from build123d import *

# Parameters (mm, degrees)
SKETCH_1_W                         = 148
SKETCH_1_H                         = 90
SKETCH_1_R                         = 11
SKETCH_1_R_2                       = 2.65
SM_BASE_FLANGE_1_DEPTH             = 4
SM_EDGE_FLANGE_1_STRIP_W           = 24
SM_EDGE_FLANGE_1_STRIP_H           = 4
SM_EDGE_FLANGE_1_STRIP_CUT_DEPTH   = 90
SM_EDGE_FLANGE_1_STRIP_2_W         = 24
SM_EDGE_FLANGE_1_STRIP_2_H         = 4
SM_EDGE_FLANGE_1_STRIP_CUT_2_DEPTH = 90
SM_EDGE_FLANGE_1_DEPTH             = 90
SM_EDGE_FLANGE_1_BEND_DEPTH        = 90
SKETCH_12_R                        = 2
CUT_EXTRUDE_1_DEPTH                = 161.031246949
FILLET_1_R                         = 10
SKETCH_13_R                        = 2
CUT_EXTRUDE_2_DEPTH                = 96.822753039


# Sheet-metal steps are written as plain solids
with BuildPart() as part:
    # Sketch 1 → Базовая кромка1 (new body)
    with BuildSketch(Plane.XY):
        Rectangle(SKETCH_1_W, SKETCH_1_H)
        Circle(SKETCH_1_R, mode=Mode.SUBTRACT)
        with Locations((20, 0)):
            Circle(SKETCH_1_R_2, mode=Mode.SUBTRACT)
        with Locations((-20, 0)):
            Circle(SKETCH_1_R_2, mode=Mode.SUBTRACT)
        with BuildLine():
            Line((-4.9, -36.5), (-4.9, -39.5))
            ThreePointArc((-4.9, -39.5), (-7, -41.6), (-9.1, -39.5))
            Line((-9.1, -39.5), (-9.1, -36.5))
            ThreePointArc((-9.1, -36.5), (-7, -34.4), (-4.9, -36.5))
        make_face(mode=Mode.SUBTRACT)
        with BuildLine():
            Line((9.1, -36.5), (9.1, -39.5))
            ThreePointArc((9.1, -39.5), (7, -41.6), (4.9, -39.5))
            Line((4.9, -39.5), (4.9, -36.5))
            ThreePointArc((4.9, -36.5), (7, -34.4), (9.1, -36.5))
        make_face(mode=Mode.SUBTRACT)
    extrude(amount=-SM_BASE_FLANGE_1_DEPTH)

    # Ребро-кромка1 strip (across the edge) → Ребро-кромка1 strip cut (cut)
    with BuildSketch(Plane(origin=(-74, 45, 0), x_dir=(1, 0, 0), z_dir=(0, -1, 0))):
        with Locations((-4, -2)):
            Rectangle(SM_EDGE_FLANGE_1_STRIP_W, SM_EDGE_FLANGE_1_STRIP_H)
    extrude(amount=SM_EDGE_FLANGE_1_STRIP_CUT_DEPTH, mode=Mode.SUBTRACT)

    # Ребро-кромка1 strip 2 (across the edge) → Ребро-кромка1 strip cut 2 (cut)
    with BuildSketch(Plane(origin=(74, -45, 0), x_dir=(-1, 0, 0), z_dir=(0, 1, 0))):
        with Locations((-4, -2)):
            Rectangle(SM_EDGE_FLANGE_1_STRIP_2_W, SM_EDGE_FLANGE_1_STRIP_2_H)
    extrude(amount=SM_EDGE_FLANGE_1_STRIP_CUT_2_DEPTH, mode=Mode.SUBTRACT)

    # Ребро-кромка1 section (across the edge) → Ребро-кромка1 (add)
    with BuildSketch(Plane(origin=(-74, 45, 0), x_dir=(1, 0, 0), z_dir=(0, -1, 0))):
        with BuildLine():
            Line((0, 4), (0, 41))
            Line((0, 41), (4, 41))
            Line((4, 41), (4, 4))
            ThreePointArc((4, 4), (5.171572875, 1.171572875), (8, 0))
            Line((8, 0), (8, -4))
            ThreePointArc((8, -4), (2.343145751, -1.656854249), (0, 4))
        make_face()
    extrude(amount=SM_EDGE_FLANGE_1_DEPTH)

    # Ребро-кромка1 section 2 (across the edge) → Ребро-кромка1 bend (add)
    with BuildSketch(Plane(origin=(74, -45, 0), x_dir=(-1, 0, 0), z_dir=(0, 1, 0))):
        with BuildLine():
            Line((0, 4), (0, 41))
            Line((0, 41), (4, 41))
            Line((4, 41), (4, 4))
            ThreePointArc((4, 4), (5.171572875, 1.171572875), (8, 0))
            Line((8, 0), (8, -4))
            ThreePointArc((8, -4), (2.343145751, -1.656854249), (0, 4))
        make_face()
    extrude(amount=SM_EDGE_FLANGE_1_BEND_DEPTH)

    # Эскиз12 → Вырез-Вытянуть1 (cut, through all)
    with BuildSketch(Plane(origin=(74, 0, 0), x_dir=(0, 0, -1), z_dir=(1, 0, 0))):
        with Locations((-31, 35)):
            Circle(SKETCH_12_R)
        with Locations((-31, -35)):
            Circle(SKETCH_12_R)
        with Locations((-31, 0)):
            Circle(SKETCH_12_R)
    extrude(amount=-CUT_EXTRUDE_1_DEPTH, mode=Mode.SUBTRACT)

    # Скругление1
    fillet_1_edges = [part.edges().sort_by_distance(p)[0] for p in [
        (72, -45, 41),
        (72, 45, 41),
        (-72, 45, 41),
        (-72, -45, 41),
    ]]
    fillet(fillet_1_edges, radius=FILLET_1_R)

    # Эскиз13 → Вырез-Вытянуть2 (cut, through all)
    with BuildSketch(Plane.XY):
        with Locations((-32, 38)):
            Circle(SKETCH_13_R)
        with Locations((32, 38)):
            Circle(SKETCH_13_R)
        with Locations((32, -38)):
            Circle(SKETCH_13_R)
        with Locations((-32, -38)):
            Circle(SKETCH_13_R)
    extrude(amount=-CUT_EXTRUDE_2_DEPTH, mode=Mode.SUBTRACT)


solid = part.part
Check sheet for the modelled part. Datum: model origin and axes. Units: mm. A direction names the side the tool comes from. Coordinates: 2 decimals unless noted, no trailing zeros. Loops run counter-clockwise (first coordinate to the right, second up) from the corner with the lowest first, then second, coordinate; pieces in that order, holes last. Notation, with made-up numbers: (38.25, 54) -> (92.25, 54) arc R33 ccw to (92.25, 90) -> close; hole circle Ø3 at (8, -21.75). An arc over 180 degrees is marked (long way). Answer in a Markdown table with one row per item.
1. Sectioned sample at B-B, the plane z = 8. Record the boundary of the cut face in (x, y).
Check values:
| item | result |
|---|---|
| outline | (-74, -45) -> (-70, -45) -> (-70, 45) -> (-74, 45) -> close; (70, -45) -> (74, -45) -> (74, 45) -> (70, 45) -> close |
2. Material ranges on line 1 along Y through (x, z) = (71.7, 31); line 2 along Y through (x, z) = (-32, -1.5); line 3 along X through (y, z) = (-32, 27), recorded low to high. Write a range as [from, to].
Check values:
| item | result |
|---|---|
| line 1 | y = [-45, -37], [-33, -2], [2, 33], [37, 45] |
| line 2 | y = [-45, -40], [-36, 36], [40, 45] |
| line 3 | x = [-74, -70], [70, 74] |
3. Go/stop test with flat-tipped pins: pin 1 (2.5 mm diameter, centred on x = 32, y = 38, fed in from -Z); pin 2 (6.5 mm diameter, centred on x = 32, y = -38, fed in from -Z); pin 3 (2.5 mm diameter, centred on y = -37.5, z = -3, fed in from -X); pin 4 (8.5 mm diameter, centred on x = 20, y = 0, fed in from +Z). Record where each tip stops, or that it passes through.
Check values:
| item | result |
|---|---|
| pin 1 | passes through |
| pin 2 | stops at z = -4 |
| pin 3 | stops at x = -71.56 |
| pin 4 | stops at z = 0 |
4. Release check for a two-part mould opening along Y. For faces 4 (the face through (-68.859, 0.63, 1.203)), 5 (the face through (7, -34.4, -2)), 6 (the face through (0, -45, -1)), 7 (the face through (71.97, 42.15, 37.99)) record: released by +Y, released by -Y, zero draft, split by the parting line, or undercut.
Check values:
| item | result |
|---|---|
| face 4 | zero draft |
| face 5 | undercut |
| face 6 | released by -Y |
| face 7 | released by +Y |
5. Access from +Z, -Z, +X, -X, +Y, -Y to the whole of each face (thin tool, end or side, straight path). Record for faces 1 (the face through (-7, -41.6, -2)), 2 (the face through (-74, 1, 22)), 3 (the face through (70, -1, 23)).
Check values:
| item | result |
|---|---|
| face 1 | +Z, -Z |
| face 2 | +Z, -Z, -X, +Y, -Y |
| face 3 | +Z, +Y, -Y |
6. Sectioned sample at D-D, the plane y = -20. Record the boundary of the cut face in (x, z).
Check values:
| item | result |
|---|---|
| outline | (-74, 4) arc R8 ccw to (-66, -4) -> (66, -4) arc R8 ccw to (74, 4) -> (74, 41) -> (70, 41) -> (70, 4) arc R4 cw to (66, 0) -> (-66, 0) arc R4 cw to (-70, 4) -> (-70, 41) -> (-74, 41) -> close |
7. Sectioned sample at A-A, the plane y = 0. Give the number of separate pieces and of enclosed holes in the cut face, then the cut area to 3 significant figures.
Check values:
| item | result |
|---|---|
| separate pieces | 6 |
| enclosed holes | 0 |
| area | 737 mm2 |
8. Sectioned sample at C-C, the plane x = 7. Record the boundary of the cut face in (y, z), then the cut area to 3 significant figures.
Check values:
| item | result |
|---|---|
| outline | (-45, -4) -> (-41.6, -4) -> (-41.6, 0) -> (-45, 0) -> close; (-34.4, -4) -> (-8.49, -4) -> (-8.49, 0) -> (-34.4, 0) -> close; (8.49, -4) -> (45, -4) -> (45, 0) -> (8.49, 0) -> close |
| area | 263 mm2 |
